from build123d import *

# Parameters (mm, degrees)
BOSS_EXTRUDE2_START     = 10
BOSS_EXTRUDE2_DEPTH     = 8
SKETCH6_R               = 1.05
CUT_EXTRUDE1_DEPTH      = 3.9
CUT_EXTRUDE1_DEPTH_BACK = 8.5
CUT_EXTRUDE2_DEPTH      = 0.8
BOSS_EXTRUDE6_DEPTH     = 1.6
SKETCH9_R               = 1.05
CUT_EXTRUDE3_DEPTH      = 9


with BuildPart() as part:
    # Sketch2 → Boss-Extrude2 (new body)
    with BuildSketch(Plane(origin=(0, 0, 0), x_dir=(1, 0, 0), z_dir=(0, 1, 0)).offset(BOSS_EXTRUDE2_START)):
        with BuildLine():
            Line((-4.663689527, 2.3), (-12, 2.3))
            Line((-12, 2.3), (-12, 0.7))
            Line((-12, 0.7), (-3.633180425, 0.7))
            ThreePointArc((-3.633180425, 0.7), (3.7, 0), (-3.633180425, -0.7))
            Line((-3.633180425, -0.7), (-12, -0.7))
            Line((-12, -0.7), (-12, -2.3))
            Line((-12, -2.3), (-4.663689527, -2.3))
            ThreePointArc((-4.663689527, -2.3), (5.2, 0), (-4.663689527, 2.3))
        make_face()
    extrude(amount=BOSS_EXTRUDE2_DEPTH)

    # Sketch6 → Cut-Extrude1 (cut, two sides)
    with BuildSketch(Plane.XY.offset(2.3)) as cut_extrude1_sk:
        with Locations((-8.331844763, 14)):
            Circle(SKETCH6_R)
    extrude(amount=CUT_EXTRUDE1_DEPTH, mode=Mode.SUBTRACT)
    extrude(cut_extrude1_sk.sketch, amount=-CUT_EXTRUDE1_DEPTH_BACK, mode=Mode.SUBTRACT)

    # Sketch7 → Cut-Extrude2 (cut)
    with BuildSketch(Plane.XY.offset(2.3)):
        Polygon((-6.331844763, 15.154700538), (-8.331844763, 16.309401077), (-10.331844763, 15.154700538), (-10.331844763, 12.845299462), (-8.331844763, 11.690598923), (-6.331844763, 12.845299462), align=None)
    extrude(amount=-CUT_EXTRUDE2_DEPTH, mode=Mode.SUBTRACT)

    # Sketch8 → Boss-Extrude6 (add)
    with BuildSketch(Plane.XZ.offset(-18)):
        with BuildLine():
            Line((0.667949192, -5.156921938), (8.076329488, -17.988613012))
            ThreePointArc((8.076329488, -17.988613012), (0, -19.718450651), (-8.076329488, -17.988613012))
            Line((-8.076329488, -17.988613012), (-0.667949192, -5.156921938))
            ThreePointArc((-0.667949192, -5.156921938), (-2.6, -4.5033321), (-4.132050808, -3.156921938))
            Line((-4.132050808, -3.156921938), (-11.540431103, -15.988613012))
            Line((-11.540431103, -15.988613012), (-14.050754094, -20.336619975))
            ThreePointArc((-14.050754094, -20.336619975), (24.718450651, 0), (-14.050754094, 20.336619975))
            Line((-14.050754094, 20.336619975), (-11.540431103, 15.988613012))
            Line((-11.540431103, 15.988613012), (-4.132050808, 3.156921938))
            ThreePointArc((-4.132050808, 3.156921938), (-2.6, 4.5033321), (-0.667949192, 5.156921938))
            Line((-0.667949192, 5.156921938), (-8.076329488, 17.988613012))
            ThreePointArc((-8.076329488, 17.988613012), (0, 19.718450651), (8.076329488, 17.988613012))
            Line((8.076329488, 17.988613012), (0.667949192, 5.156921938))
            ThreePointArc((0.667949192, 5.156921938), (2.6, 4.5033321), (4.132050808, 3.156921938))
            Line((4.132050808, 3.156921938), (11.540431103, 15.988613012))
            ThreePointArc((11.540431103, 15.988613012), (17.076679187, 9.859225326), (19.616760591, 2))
            Line((19.616760591, 2), (4.8, 2))
            ThreePointArc((4.8, 2), (5.2, 0), (4.8, -2))
            Line((4.8, -2), (19.616760591, -2))
            ThreePointArc((19.616760591, -2), (17.076679187, -9.859225326), (11.540431103, -15.988613012))
            Line((11.540431103, -15.988613012), (4.132050808, -3.156921938))
            ThreePointArc((4.132050808, -3.156921938), (2.6, -4.5033321), (0.667949192, -5.156921938))
        make_face()
    extrude(amount=BOSS_EXTRUDE6_DEPTH)

    # Sketch9 → Cut-Extrude3 (cut, through all)
    with BuildSketch(Plane(origin=(0, 18, 0), x_dir=(1, 0, 0), z_dir=(0, 1, 0))):
        with Locations((-7.62, 21.59)):
            Circle(SKETCH9_R)
        with Locations((-10.16, -20.32)):
            Circle(SKETCH9_R)
        with Locations((10.16, -20.32)):
            Circle(SKETCH9_R)
        with Locations((21.59, -6.35)):
            Circle(SKETCH9_R)
    extrude(amount=-CUT_EXTRUDE3_DEPTH, mode=Mode.SUBTRACT)


solid = part.part
The listing builds one solid part. Answer for the finished solid, in the listing's coordinates (mm). A direction names the side the tool comes from. Give positions to 0.01 mm unless a question says otherwise; leave off trailing zeros. Order: outer loops, then holes, each group sorted by start corner. A loop starts at its lowest first (then second) coordinate and runs counter-clockwise, first axis right, second up. Notation, with made-up numbers: (1, 80.25) - (28, 80.25) arc R29 cw to (28, 115.25) - close; hole circle Ø7 at (-38, 38.25). An arc over 180 degrees is marked (long way). Answer as CSV lines item,"result".
Q1. A cutting plane is placed at B-B, the plane x = 0. Determine the outline of the cut face in (y, z).
Answer key:
outline,"(10, -5.2) - (18, -5.2) - (18, -3.7) - (10, -3.7) - close; (10, 3.7) - (18, 3.7) - (18, 5.2) - (10, 5.2) - close; (16.4, -24.72) - (18, -24.72) - (18, -19.72) - (16.4, -19.72) - close; (16.4, 19.72) - (18, 19.72) - (18, 24.72) - (16.4, 24.72) - close"
Q2. A cutting plane is placed at A-A, the plane y = 14. Determine the outline of the cut face in (x, z), and give its area (3 significant figures).
Answer key:
outline,"(-12, -2.3) - (-9.38, -2.3) - (-9.38, -0.7) - (-12, -0.7) - close; (-12, 0.7) - (-9.38, 0.7) - (-9.38, 1.5) - (-10.33, 1.5) - (-10.33, 2.3) - (-12, 2.3) - close; (-7.28, -2.3) - (-4.66, -2.3) arc R5.2 ccw (long way) to (-4.66, 2.3) - (-6.33, 2.3) - (-6.33, 1.5) - (-7.28, 1.5) - (-7.28, 0.7) - (-3.63, 0.7) arc R3.7 cw (long way) to (-3.63, -0.7) - (-7.28, -0.7) - close"
area,"54.1 mm^2"
Q3. Each of these flat-tipped pins is pushed along its axis until it touches: pin 1 Ø1.3 at (x, y) = (14, 17) entering from +Z; pin 2 Ø2 at (x, y) = (-9, 13) entering from -Z; pin 3 Ø1.3 at (y, z) = (15, -1.5) entering from -X. Where does it stop, or does it pass through?
Answer key:
pin 1,"stops at z = 20.8"
pin 2,"stops at z = -2.3"
pin 3,"stops at x = -12"
Q4. A cutting plane is placed at C-C, the plane z = 6.35. Determine the outline of the cut face in (x, y).
Answer key:
outline,"(-5.98, 16.4) - (-1.36, 16.4) - (-1.36, 18) - (-5.98, 18) - close; (1.36, 16.4) - (5.98, 16.4) - (5.98, 18) - (1.36, 18) - close; (18.67, 16.4) - (20.54, 16.4) - (20.54, 18) - (18.67, 18) - close; (22.64, 16.4) - (23.89, 16.4) - (23.89, 18) - (22.64, 18) - close"
Q5. A cutting plane is placed at D-D, the plane z = 14.5. Determine the outline of the cut face in (x, y).
Answer key:
outline,"(-10.68, 16.4) - (-6.06, 16.4) - (-6.06, 18) - (-10.68, 18) - close; (6.06, 16.4) - (10.68, 16.4) - (10.68, 18) - (6.06, 18) - close; (13.36, 16.4) - (20.02, 16.4) - (20.02, 18) - (13.36, 18) - close"
Q6. Straight lines are drawn through the part: L1, parallel to Z at x = -8, y = 12; L2, parallel to Z at x = -10.16, y = 17.3; L3, parallel to Y at x = 19.5, z = -12. For each, find the intervals that lie inside material, in ascending order.
Answer key:
L1,"z = -2.3 to -0.7, 0.7 to 1.5"
L2,"z = -22.53 to -13.6, -2.3 to -0.7, 0.7 to 2.3, 13.6 to 19.27, 21.37 to 22.53"
L3,"y = 16.4 to 18"
Q7. Determine the mould class of faces 5 (the face through (24.707, 17.211, -0.753)), 6 (the face through (-7.346, 12.26, 1.906)), 7 (the face through (4.32, 17.21, -11.48)) for opening direction Z: pulls with the +Z half, pulls with the -Z half, needs draft (parallel to the pull), parting line crosses it, or undercut.
Answer key:
face 5,"parting line crosses it"
face 6,"needs draft"
face 7,"undercut"
Q8. Which of the six approach directions +Z, -Z, +X, -X, +Y, -Y give full straight-line access (tool end or side, diameter ignored) to faces 1 (the face through (-4, 10, -1)), 2 (the face through (17.135, 17.211, -9.758)), 3 (the face through (-12, 14, 1)), 4 (the face through (-7.318, 15.724, 1.906))?
Answer key:
face 1,"+Z, -Z, +X, -X, -Y"
face 2,"+Y, -Y"
face 3,"-X, +Y, -Y"
face 4,"+Z"
